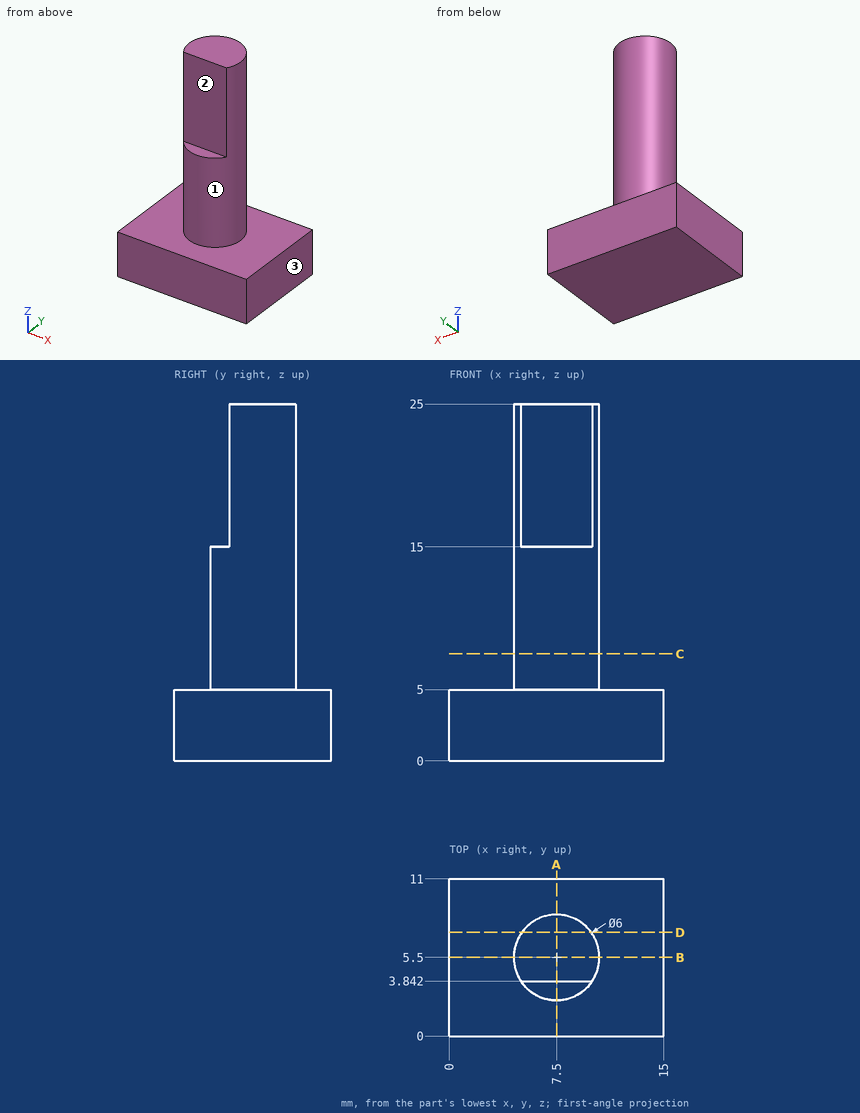
For this review, use the dimensioned drawing (mm, ordinates from the lowest corner) and the shaded views. A direction names the side the tool comes from. Round coordinates to 2 decimals unless told otherwise and drop trailing zeros. Write each loop counter-clockwise with the first axis right and the second up, starting at its lowest first coordinate (ties: lowest second). Pieces come first, ordered by that corner, then holes. Notation, with made-up numbers: M 74,50 L 119,50 A23 cw 119,79 Z; hole C -24.5,11.5 d5. An arc over 180 degrees is marked long. Write item = value, one per line. Start each with the question number.
(1) We need section C-C (z = 7.5). Give the boundary of the cut face in (x, y).
(2) We need section B-B (y = 5.5). Give the boundary of the cut face in (x, z).
(3) For line 1 along Z through (x, y) = (9, 3.75); line 2 along Z through (x, y) = (4.25, 9.75); line 3 along X through (y, z) = (4.75, 12) (1 decimal), list the stretches that pass through material, from the lowest coordinate up.
(4) Clearance check with flat-ended pins moving along their axes: pin 1 Ø1.5 at (x, z) = (6, 16.5) entering from -Y; pin 2 Ø8 at (x, z) = (12.5, 10.5) entering from -Y; pin 3 Ø1 at (y, z) = (7, 9.5) entering from +X. State where each tip first meets the part, or that it passes through.
(5) For the marked faces 1, 2 and 3, list the 3-axis set-ups (+Z, -Z, +X, -X, +Y, -Y) from which the entire face can be reached by the end or side of a thin tool; tool diameter is ignored.
(6) We need section A-A (x = 7.5). Give the boundary of the cut face in (y, z).
(7) We need section D-D (y = 7.25). Give the boundary of the cut face in (x, z).
Results found:
q1.outline = C 7.5,5.5 d6
q2.outline = M 0,0 L 15,0 L 15,5 L 10.5,5 L 10.5,25 L 4.5,25 L 4.5,5 L 0,5 Z
q3.line_1 = 0 to 15
q3.line_2 = 0 to 5
q3.line_3 = 4.6 to 10.4
q4.pin_1 = 3.84
q4.pin_2 = 2.67
q4.pin_3 = 10.33
q5.face_1 = +Z
q5.face_2 = +Z, +X, -X, -Y
q5.face_3 = +Z, -Z, +X, +Y, -Y
q6.outline = M 0,0 L 11,0 L 11,5 L 8.5,5 L 8.5,25 L 3.84,25 L 3.84,15 L 2.5,15 L 2.5,5 L 0,5 Z
q7.outline = M 0,0 L 15,0 L 15,5 L 9.94,5 L 9.94,25 L 5.06,25 L 5.06,5 L 0,5 Z
